Read the model definition and answer for the solid it produces. Units are mm, in the model's axes. Face numbers are marked on the shaded views. A direction names the side the tool comes from. Give positions to 0.01 mm unless a question says otherwise; leave off trailing zeros. Write each loop counter-clockwise with the first axis right and the second up, starting at its lowest first coordinate (ties: lowest second). Pieces come first, ordered by that corner, then holes. Notation, with made-up numbers: (82, -29) -> (97, -29) arc R25 ccw to (97, -2) -> close; hole circle Ø9 at (11, 61). An arc over 180 degrees is marked (long way). Use a Markdown table: item, result.
from build123d import *

# Parameters (mm, degrees)
SKETCH1_R               = 2
BOSS_EXTRUDE1_DEPTH     = 8
SKETCH1_3_R             = 3.55
SKETCH1_3_R_2           = 2
BOSS_EXTRUDE2_DEPTH     = 2
SKETCH2_R               = 4.7
BOSS_EXTRUDE3_DEPTH     = 8
SKETCH3_R               = 3.15
CUT_EXTRUDE1_DEPTH      = 20.188017094
CUT_EXTRUDE1_DEPTH_BACK = 7
CHAMFER1_SIZE           = 3.3
CHAMFER1_SIZE2          = 0.884232335
SKETCH4_W               = 2.2
SKETCH4_H               = 7
CUT_EXTRUDE2_DEPTH      = 13.007497658
CUT_EXTRUDE2_DEPTH_BACK = 13.007497658
FILLET1_R               = 1


with BuildPart() as part:
    # Sketch1 → Boss-Extrude1 (new body)
    with BuildSketch(Plane(origin=(0, 0, 0), x_dir=(1, 0, 0), z_dir=(0, 1, 0))):
        with Locations(Location((0, 0, 0), (0, 0, 270))):
            Circle(SKETCH1_R)
    extrude(amount=-BOSS_EXTRUDE1_DEPTH)

    # Sketch1_3 → Boss-Extrude2 (add)
    with BuildSketch(Plane(origin=(0, 0, 0), x_dir=(1, 0, 0), z_dir=(0, 1, 0))):
        with Locations(Location((0, 0, 0), (0, 0, 270))):
            Circle(SKETCH1_3_R)
        with Locations(Location((0, 0, 0), (0, 0, 270))):
            Circle(SKETCH1_3_R_2, mode=Mode.SUBTRACT)
        with Locations(Location((0, 0, 0), (0, 0, 270))):
            Circle(SKETCH1_3_R_2)
    extrude(amount=BOSS_EXTRUDE2_DEPTH)

    # Sketch2 → Boss-Extrude3 (add)
    with BuildSketch(Plane(origin=(0, 2, 0), x_dir=(1, 0, 0), z_dir=(0, 1, 0))):
        with Locations(Location((0, 0, 0), (0, 0, 270))):
            Circle(SKETCH2_R)
    extrude(amount=BOSS_EXTRUDE3_DEPTH)

    # Sketch3 → Cut-Extrude1 (cut, two sides)
    with BuildSketch(Plane(origin=(0, 10, 0), x_dir=(1, 0, 0), z_dir=(0, 1, 0))) as cut_extrude1_sk:
        with Locations(Location((0, 0, 0), (0, 0, 90))):
            Circle(SKETCH3_R)
    extrude(amount=CUT_EXTRUDE1_DEPTH, mode=Mode.SUBTRACT)
    extrude(cut_extrude1_sk.sketch, amount=-CUT_EXTRUDE1_DEPTH_BACK, mode=Mode.SUBTRACT)

    # Chamfer1
    chamfer1_edges = [part.edges().sort_by_distance(p)[0] for p in [
        (0, 10, 3.15),
    ]]
    chamfer1_side = [part.faces().sort_by_distance(p)[0] for p in [
        (0, 6.5, 3.15),
    ]]
    chamfer(chamfer1_edges, length=CHAMFER1_SIZE, length2=CHAMFER1_SIZE2, reference=chamfer1_side[0])

    # Sketch4 → Cut-Extrude2 (cut, two sides)
    with BuildSketch(Plane.XY) as cut_extrude2_sk:
        with Locations((0, 6.5)):
            Rectangle(SKETCH4_W, SKETCH4_H)
    extrude(amount=CUT_EXTRUDE2_DEPTH, mode=Mode.SUBTRACT)
    extrude(cut_extrude2_sk.sketch, amount=-CUT_EXTRUDE2_DEPTH_BACK, mode=Mode.SUBTRACT)

    # Fillet1
    fillet1_edges = [part.edges().sort_by_distance(p)[0] for p in [
        (1.1, 3, 3.760579146),
        (1.1, 3, -3.760579146),
        (-1.1, 3, -3.760579146),
        (-1.1, 3, 3.760579146),
    ]]
    fillet(fillet1_edges, radius=FILLET1_R)


solid = part.part
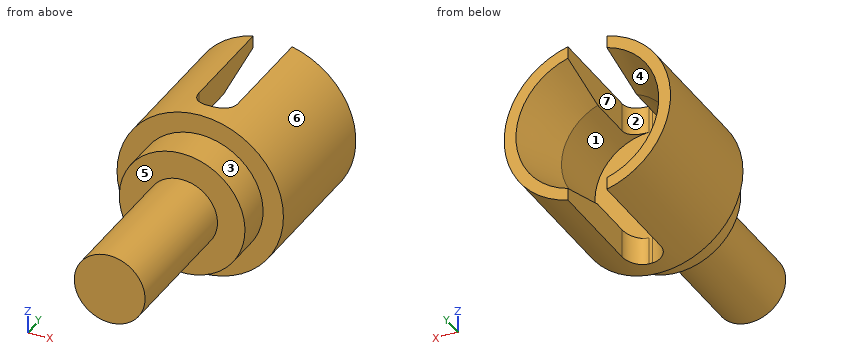
Item 1: For a pull along Z with two mould halves and no side action, classify the marked faces 1, 2 and 3 as +Z half, -Z half, draft (parallel to the pull), parting line (faces both ways), or undercut.
Return value:
| item | result |
|---|---|
| face 1 | undercut |
| face 2 | draft |
| face 3 | parting line |
Item 2: A cutting plane is placed at B-B (y = 8.25). Give the vertices of the cut face in (x, z), then the cut area to 3 significant figures.
Return value:
| item | result |
|---|---|
| outline | (-1.1, -4.57) -> (-1.1, -3.39) arc R3.57 cw to (-1.1, 3.39) -> (-1.1, 4.57) arc R4.7 ccw to start; (1.1, -4.57) arc R4.7 ccw to (1.1, 4.57) -> (1.1, 3.39) arc R3.57 cw to (1.1, -3.39) -> close |
| area | 24.4 mm^2 |
Item 3: A cutting plane is placed at A-A (z = 0). Give the vertices of the cut face in (x, y).
Return value:
| item | result |
|---|---|
| outline | (-4.7, 2) -> (-3.55, 2) -> (-3.55, 0) -> (-2, 0) -> (-2, -8) -> (2, -8) -> (2, 0) -> (3.55, 0) -> (3.55, 2) -> (4.7, 2) -> (4.7, 10) -> (4.03, 10) -> (3.15, 6.7) -> (3.15, 3) -> (-3.15, 3) -> (-3.15, 6.7) -> (-4.03, 10) -> (-4.7, 10) -> close |
Item 4: A cutting plane is placed at C-C (x = 4.25). Give the vertices of the cut face in (y, z), then the cut area to 3 significant figures.
Return value:
| item | result |
|---|---|
| outline | (2, -2.01) -> (10, -2.01) -> (10, 2.01) -> (2, 2.01) -> close |
| area | 32.1 mm^2 |
Item 5: A cutting plane is placed at D-D (y = -4.5). Give the vertices of the cut face in (x, z).
Return value:
| item | result |
|---|---|
| outline | circle Ø4 at (0, 0) |
Item 6: Straight lines are drawn through the part: line 1 along Y through (x, z) = (-0.75, 3); line 2 along Z through (x, y) = (2, 6); line 3 along Y through (x, z) = (-1.25, -0.5). For each, find the intervals that lie inside material, in ascending order. Write a range as [from, to].
Return value:
| item | result |
|---|---|
| line 1 | [0, 3] |
| line 2 | [-4.25, -2.43], [2.43, 4.25] |
| line 3 | [-8, 3] |
Item 7: Each of these flat-tipped pins is pushed along its axis until it touches: P1, Ø1.3, axis at y = 7.5, z = -3.5, coming from the -X side; P2, Ø0.5, axis at y = 5.5, z = 4, coming from the +X side; P3, Ø1.5, axis at y = 3, z = 3.5, coming from the -X side. Where does it stop, or does it pass through?
Return value:
| item | result |
|---|---|
| P1 | x = -3.74 |
| P2 | x = 2.83 |
| P3 | x = -3.81 |
Item 8: A tool of negligible diameter and unlimited length cuts with its end or side. For the marked faces 4, 5, 6 and 7, from which of +Z, -Z, +X, -X, +Y, -Y can it reach the whole face along a straight path? Write none if from no direction.
Return value:
| item | result |
|---|---|
| face 4 | +Y |
| face 5 | -Y |
| face 6 | +Y, -Y |
| face 7 | +Z, -Z, +Y |
